from build123d import *

# Parameters (mm, degrees)
BOSS_EXTRUDE1_DEPTH = 30.48
SKETCH2_R           = 4.2545
BOSS_EXTRUDE2_DEPTH = 2.54
SKETCH3_R           = 1.016
BOSS_EXTRUDE3_DEPTH = 1.27
SKETCH4_R           = 3.048
BOSS_EXTRUDE4_DEPTH = 1.5875
SKETCH5_R           = 1.0287
BOSS_EXTRUDE5_DEPTH = 9.8552
SKETCH6_R           = 1.27
CUT_EXTRUDE1_DEPTH  = 3.175


with BuildPart() as part:
    # Sketch1 → Boss-Extrude1 (new body)
    with BuildSketch(Plane.XY):
        with BuildLine():
            Line((-7.12333026, -9.2075), (7.12333026, -9.2075))
            ThreePointArc((7.12333026, -9.2075), (7.679816379, -9.102266788), (8.159451026, -8.8011))
            ThreePointArc((8.159451026, -8.8011), (12.0015, 0), (8.159451026, 8.8011))
            ThreePointArc((8.159451026, 8.8011), (7.679816379, 9.102266788), (7.12333026, 9.2075))
            Line((7.12333026, 9.2075), (-7.12333026, 9.2075))
            ThreePointArc((-7.12333026, 9.2075), (-7.679816379, 9.102266788), (-8.159451026, 8.8011))
            ThreePointArc((-8.159451026, 8.8011), (-12.0015, 0), (-8.159451026, -8.8011))
            ThreePointArc((-8.159451026, -8.8011), (-7.679816379, -9.102266788), (-7.12333026, -9.2075))
        make_face()
    extrude(amount=BOSS_EXTRUDE1_DEPTH)

    # Sketch2 → Boss-Extrude2 (add)
    with BuildSketch(Plane.XY.offset(30.48)):
        with Locations(Location((0, 0, 0), (0, 0, 180))):  # turned: the seam where the file's is
            Circle(SKETCH2_R)
    extrude(amount=BOSS_EXTRUDE2_DEPTH)

    # Sketch3 → Boss-Extrude3 (add)
    with BuildSketch(Plane.XY.offset(33.02)):
        Circle(SKETCH3_R)
    extrude(amount=BOSS_EXTRUDE3_DEPTH)

    # Sketch4 → Boss-Extrude4 (add)
    with BuildSketch(Plane(origin=(0, 0, 0), x_dir=(-1, 0, 0), z_dir=(0, 0, -1))):
        Circle(SKETCH4_R)
    extrude(amount=BOSS_EXTRUDE4_DEPTH)

    # Sketch5 → Boss-Extrude5 (add)
    with BuildSketch(Plane(origin=(0, 0, -1.5875), x_dir=(-1, 0, 0), z_dir=(0, 0, -1))):
        Circle(SKETCH5_R)
    extrude(amount=BOSS_EXTRUDE5_DEPTH)

    # Sketch6 → Cut-Extrude1 (cut)
    with BuildSketch(Plane(origin=(0, 9.2075, 0), x_dir=(1, 0, 0), z_dir=(0, 1, 0))):
        with Locations(Location((4.699, -27.94, 0), (0, 0, 270))):  # turned: the seam where the file's is
            Circle(SKETCH6_R)
        with Locations(Location((-4.699, -27.94, 0), (0, 0, 270))):  # turned: the seam where the file's is
            Circle(SKETCH6_R)
    extrude(amount=-CUT_EXTRUDE1_DEPTH, mode=Mode.SUBTRACT)


solid = part.part
The model under review builds one solid part; all positions refer to its coordinate system, in mm. A direction names the side the tool comes from. Give positions to 0.01 mm unless a question says otherwise; leave off trailing zeros. Order: outer loops, then holes, each group sorted by start corner. A loop starts at its lowest first (then second) coordinate and runs counter-clockwise, first axis right, second up. Notation, with made-up numbers: M 61,-34 L 86,-34 A14 ccw 86,-18 Z; hole C -33,-26 d7. An arc over 180 degrees is marked long. Use one line per item in the form item = value. Start each with the question number.
Item 1: We need section D-D on y = 8. Give the boundary of the cut face in (x, z), plus the area to 3 significant figures.
Item 2: To check wall thickness, follow line 1 along X through (y, z) = (6.8, 27.94); line 2 along Z through (x, y) = (-10, -6.25); line 3 along X through (y, z) = (0, 12). State the ranges of each line that lie inside material, in increasing order. Write a range as from..to.
Item 3: For faces 1 (the flat face through (5, 6.032, 28)), 2 (the flat face through (-3, 2, 0)), 3 (the cylindrical face through (-7.672, 9.105, 15.027)), 4 (the flat face through (-1, 1, 33.02)), 5 (the flat face through (0, -9.208, 15)), list the 3-axis set-ups (+Z, -Z, +X, -X, +Y, -Y) from which the entire face can be reached by the end or side of a thin tool; tool diameter is ignored.
Item 4: We need section A-A on y = 0. Give the boundary of the cut face in (x, z), plus the area to 3 significant figures.
Item 5: We need section C-C on x = 0. Give the boundary of the cut face in (y, z).
Item 6: We need section B-B on z = 25. Give the boundary of the cut face in (x, y), plus the area to 3 significant figures.
Item 7: Insertion check: pin 1 Ø1.5 at (x, y) = (-0.5, -3.5) entering from +Z; pin 2 Ø1.5 at (x, y) = (-9, -5) entering from -Z; pin 3 Ø4 at (y, z) = (4, 9.5) entering from +X. Each pin has a flat end and moves straight along its axis. Give the tip position at first contact, or say it passes through.
Item 8: The part is to be moulded in two halves that separate along X. For faces 6 (the cylindrical face through (4.75, 7.64, 26.67)), 7 (the flat face through (0, 0, -11.443)), 8 (the cylindrical face through (12, 0, 15)), say which applies: pulls with the +X half, pulls with the -X half, needs draft (parallel to the pull), parting line crosses it, or undercut.
Completed:
q1.outline = M -8.95,0 L 8.95,0 L 8.95,30.48 L -8.95,30.48 Z; hole C -4.7,27.94 d2.54; hole C 4.7,27.94 d2.54
q1.area = 535 mm²
q2.line_1 = -9.89..-5.97, -3.43..3.43, 5.97..9.89
q2.line_2 = 0..30.48
q2.line_3 = -12..12
q3.face_1 = +Y
q3.face_2 = -Z
q3.face_3 = +Z, -Z, -X, +Y
q3.face_4 = +Z
q3.face_5 = +Z, -Z, +X, -X, -Y
q4.outline = M -12,0 L -3.05,0 L -3.05,-1.59 L -1.03,-1.59 L -1.03,-11.44 L 1.03,-11.44 L 1.03,-1.59 L 3.05,-1.59 L 3.05,0 L 12,0 L 12,30.48 L 4.25,30.48 L 4.25,33.02 L 1.02,33.02 L 1.02,34.29 L -1.02,34.29 L -1.02,33.02 L -4.25,33.02 L -4.25,30.48 L -12,30.48 Z
q4.area = 786 mm²
q5.outline = M -9.21,0 L -3.05,0 L -3.05,-1.59 L -1.03,-1.59 L -1.03,-11.44 L 1.03,-11.44 L 1.03,-1.59 L 3.05,-1.59 L 3.05,0 L 9.21,0 L 9.21,30.48 L 4.25,30.48 L 4.25,33.02 L 1.02,33.02 L 1.02,34.29 L -1.02,34.29 L -1.02,33.02 L -4.25,33.02 L -4.25,30.48 L -9.21,30.48 Z
q6.outline = M -8.16,-8.8 A1.52 ccw -7.12,-9.21 L 7.12,-9.21 A1.52 ccw 8.16,-8.8 A12 ccw 8.16,8.8 A1.52 ccw 7.12,9.21 L -7.12,9.21 A1.52 ccw -8.16,8.8 A12 ccw Z
q6.area = 394 mm²
q7.pin_1 = 33.02
q7.pin_2 = 0
q7.pin_3 = 11.83
q8.face_6 = undercut
q8.face_7 = needs draft
q8.face_8 = pulls with the +X half
